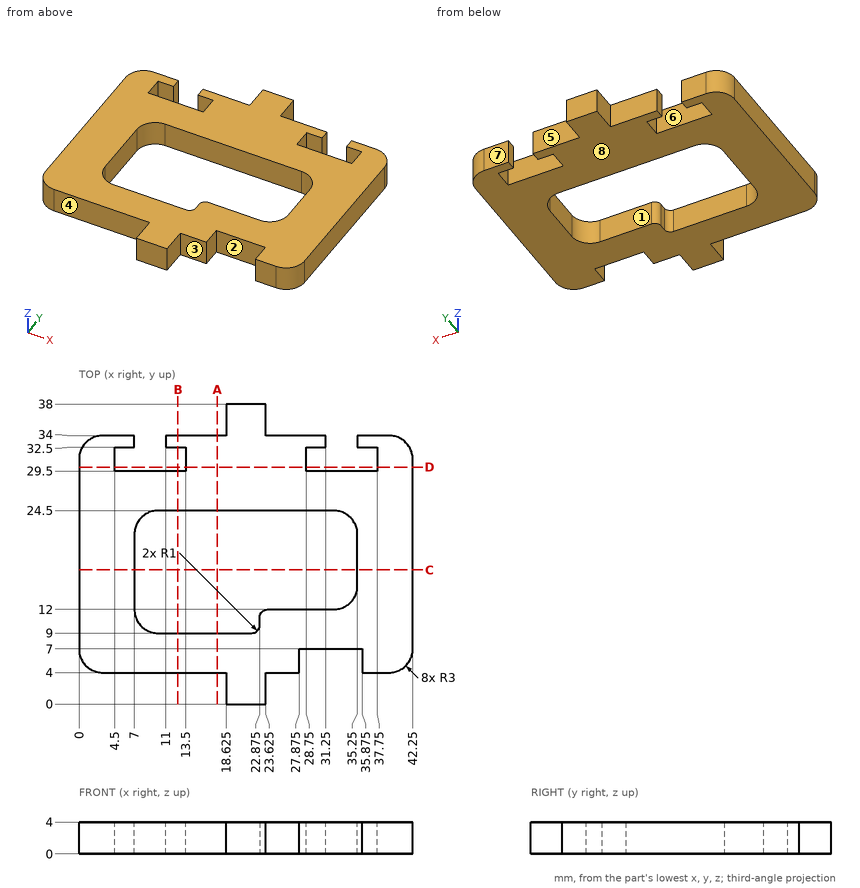
Geometry check sheet. Reference: drawing and pictorial views, mm from the part's lowest x, y, z. A direction names the side the tool comes from. Round coordinates to 2 decimals unless told otherwise and drop trailing zeros. Order: outer loops, then holes, each group sorted by start corner. A loop starts at its lowest first (then second) coordinate and runs counter-clockwise, first axis right, second up. Notation, with made-up numbers: M 47.5,59.25 L 96.5,59.25 A17 ccw 96.5,66.25 Z; hole C 29.5,62.25 d6. An arc over 180 degrees is marked long. Write item = value, one per line.
Q1. Set-up check for the marked faces 1, 2, 3, 4 and 5: record each of +Z, -Z, +X, -X, +Y, -Y from which the full face is reachable in a straight line by a thin tool's end or side.
Answer block:
face_1 = +Z, -Z
face_2 = +Z, -Z, -Y
face_3 = +Z, -Z, +X, -Y
face_4 = +Z, -Z, -X, -Y
face_5 = +Z, -Z, +X, +Y
Q2. Release check for a two-part mould opening along Y. For the marked faces 6, 7 and 8 record: released by +Y, released by -Y, zero draft, split by the parting line, or undercut.
Answer block:
face_6 = undercut
face_7 = released by +Y
face_8 = zero draft
Q3. Section check A-A (x = 17.5). Enter the section's corners in (y, z).
Answer block:
outline = M 4,0 L 9,0 L 9,4 L 4,4 Z; M 24.5,0 L 34,0 L 34,4 L 24.5,4 Z
Q4. Section check D-D (y = 30). Enter the section's corners in (x, z), plus the area to 3 significant figures.
Answer block:
outline = M 0,0 L 4.5,0 L 4.5,4 L 0,4 Z; M 13.5,0 L 28.75,0 L 28.75,4 L 13.5,4 Z; M 37.75,0 L 42.25,0 L 42.25,4 L 37.75,4 Z
area = 97.0 mm^2
Q5. Depth check by flat-ended pin: pin 1 Ø1.5 at (y, z) = (5, 2.5) entering from -X; pin 2 Ø1.5 at (y, z) = (14.5, 2) entering from -X; pin 3 Ø0.8 at (y, z) = (33, 2.5) entering from +X; pin 4 Ø1.7 at (x, z) = (38, 2) entering from -Y. Enter the tip coordinate at first touch or a pass-through.
Answer block:
pin_1 = 0.27
pin_2 = 0
pin_3 = 41.79
pin_4 = 4
Q6. Section check B-B (x = 12.5). Enter the section's corners in (y, z).
Answer block:
outline = M 4,0 L 9,0 L 9,4 L 4,4 Z; M 24.5,0 L 29.5,0 L 29.5,4 L 24.5,4 Z; M 32.5,0 L 34,0 L 34,4 L 32.5,4 Z
Q7. Scan lines: line 1 (Y direction, x = 31, z = 2.85); line 2 (Y direction, x = 11.5, z = 2.2); line 3 (Y direction, x = 26, z = 3.65). Record each from-to range of solid material in increasing order.
Answer block:
line_1 = 7 to 12, 24.5 to 29.5, 32.5 to 34
line_2 = 4 to 9, 24.5 to 29.5, 32.5 to 34
line_3 = 4 to 12, 24.5 to 34
Q8. Section check C-C (y = 17). Enter the section's corners in (x, z).
Answer block:
outline = M 0,0 L 7,0 L 7,4 L 0,4 Z; M 35.25,0 L 42.25,0 L 42.25,4 L 35.25,4 Z
